from build123d import *

# Parameters (mm, degrees)
CYLINDER001_R          = 0.75
CYLINDER001_DEPTH      = 10
CYLINDER001_ROLL_ANGLE = 90
CYLINDER002_R          = 0.75
CYLINDER002_DEPTH      = 10
CYLINDER002_ROLL_ANGLE = 90
CYLINDER_R             = 15
CYLINDER_DEPTH         = 20
CYLINDER_ROLL_ANGLE    = 90
BOX001_W               = 8
BOX001_H               = 9
BOX001_DEPTH           = 40
BOX002_W               = 8
BOX002_H               = 9
BOX002_DEPTH           = 40
BOX_W                  = 120
BOX_H                  = 20
BOX_DEPTH              = 40


with BuildPart() as zylinder001:
    # Cylinder001 → Cylinder001 (new body)
    with BuildSketch(Plane.XY):
        Circle(CYLINDER001_R)
    extrude(amount=CYLINDER001_DEPTH)


with BuildPart() as zylinder001_1:
    # Cylinder001 roll: moved
    add(zylinder001.part.rotate(Axis((0, 0, 0), (1, 0, 0)), CYLINDER001_ROLL_ANGLE))


with BuildPart() as zylinder001_2:
    # Cylinder001 placement: moved
    add(zylinder001_1.part.moved(Location((0, 10, 20))))


with BuildPart() as zylinder002:
    # Cylinder002 → Cylinder002 (new body)
    with BuildSketch(Plane.XY):
        Circle(CYLINDER002_R)
    extrude(amount=CYLINDER002_DEPTH)


with BuildPart() as zylinder002_1:
    # Cylinder002 roll: moved
    add(zylinder002.part.rotate(Axis((0, 0, 0), (1, 0, 0)), CYLINDER002_ROLL_ANGLE))


with BuildPart() as zylinder002_2:
    # Cylinder002 placement: moved
    add(zylinder002_1.part.moved(Location((50, 10, 20))))


with BuildPart() as zylinder:
    # Cylinder → Cylinder (new body)
    with BuildSketch(Plane.XY):
        Circle(CYLINDER_R)
    extrude(amount=CYLINDER_DEPTH)


with BuildPart() as zylinder_1:
    # Cylinder roll: moved
    add(zylinder.part.rotate(Axis((0, 0, 0), (1, 0, 0)), CYLINDER_ROLL_ANGLE))


with BuildPart() as zylinder_2:
    # Cylinder placement: moved
    add(zylinder_1.part.moved(Location((25, 20, 20))))


with BuildPart() as fusion001:
    # Fusion001 base: copy of Zylinder
    add(zylinder_2.part)

    # Fusion001: union Zylinder001, Zylinder002
    add(zylinder001_2.part)
    add(zylinder002_2.part)


with BuildPart() as cube001:
    # Box001 → Box001 (new body)
    with BuildSketch(Plane(origin=(-1, 8, 0), x_dir=(1, 0, 0), z_dir=(0, 0, 1))):
        with Locations((4, 4.5)):
            Rectangle(BOX001_W, BOX001_H)
    extrude(amount=BOX001_DEPTH)


with BuildPart() as cube002:
    # Box002 → Box002 (new body)
    with BuildSketch(Plane(origin=(103, 8, 0), x_dir=(1, 0, 0), z_dir=(0, 0, 1))):
        with Locations((4, 4.5)):
            Rectangle(BOX002_W, BOX002_H)
    extrude(amount=BOX002_DEPTH)


with BuildPart() as fusion002:
    # Fusion base: copy of Zylinder
    add(zylinder_2.part)

    # Fusion: union Zylinder001, Zylinder002
    add(zylinder001_2.part)
    add(zylinder002_2.part)


with BuildPart() as fusion002_1:
    # Fusion placement: moved
    add(fusion002.part.moved(Location((60, 0, 0))))

    # Fusion002: union Fusion001, Cube001, Cube002
    add(fusion001.part)
    add(cube001.part)
    add(cube002.part)


with BuildPart() as motorhalterung:
    # Box → Box (new body)
    with BuildSketch(Plane(origin=(-5, 0, 0), x_dir=(1, 0, 0), z_dir=(0, 0, 1))):
        with Locations((60, 10)):
            Rectangle(BOX_W, BOX_H)
    extrude(amount=BOX_DEPTH)

    # Cut: cut Fusion002
    add(fusion002_1.part, mode=Mode.SUBTRACT)


solid = motorhalterung.part
Verification items for the finished model (mm, model axes). A direction names the side the tool comes from. Coordinates: 2 decimals unless noted, no trailing zeros. Loops run counter-clockwise (first coordinate to the right, second up) from the corner with the lowest first, then second, coordinate; pieces in that order, holes last. Notation, with made-up numbers: (-31.75, -30) -> (25.25, -30) arc R28 cw to (25.25, 7) -> close; hole circle Ø9 at (58, 81). An arc over 180 degrees is marked (long way). Answer as CSV lines item,"result".
1) Cross-section at B-B, the plane z = 25.5. Record the cut outline in (x, y), then the cut area to 3 significant figures.
Found:
outline,"(-5, 0) -> (11.04, 0) -> (11.04, 20) -> (-5, 20) -> close; (38.96, 0) -> (71.04, 0) -> (71.04, 20) -> (38.96, 20) -> close; (98.96, 0) -> (115, 0) -> (115, 20) -> (98.96, 20) -> close; hole (-1, 8) -> (7, 8) -> (7, 17) -> (-1, 17) -> close; hole (103, 8) -> (111, 8) -> (111, 17) -> (103, 17) -> close"
area,"1,140 mm2"
2) Thickness scan on L1, parallel to Z at x = 25, y = 9.75; L2, parallel to X at y = 4, z = 17; L3, parallel to X at y = 3, z = 16. Record the ranges inside material, lowest first. Write a range as from..to.
Found:
L1,"z = 0..5, 35..40"
L2,"x = -5..10.3, 39.7..70.3, 99.7..115"
L3,"x = -5..10.54, 39.46..70.54, 99.46..115"
3) Cross-section at A-A, the plane y = 12.75. Record the cut outline in (x, z), then the cut area to 3 significant figures.
Found:
outline,"(-5, 0) -> (-1, 0) -> (-1, 40) -> (-5, 40) -> close; (7, 0) -> (103, 0) -> (103, 40) -> (7, 40) -> close; (111, 0) -> (115, 0) -> (115, 40) -> (111, 40) -> close; hole circle Ø30 at (25, 20); hole circle Ø30 at (85, 20)"
area,"2,750 mm2"
4) Tool access check on faces 5 (the flat face through (3, 8, 20)), 6 (the flat face through (115, 10, 20)). Record the directions out of +Z, -Z, +X, -X, +Y, -Y that give a thin tool (end or side, any length) a straight path to the whole face; none if there is none.
Found:
face 5,"+Z, -Z"
face 6,"+Z, -Z, +X, +Y, -Y"
5) Cross-section at C-C, the plane x = 85. Record the cut outline in (y, z), then the cut area to 3 significant figures.
Found:
outline,"(0, 0) -> (20, 0) -> (20, 5) -> (0, 5) -> close; (0, 35) -> (20, 35) -> (20, 40) -> (0, 40) -> close"
area,"200 mm2"
6) Depth check by flat-ended pin: pin 1 (12 mm diameter, centred on x = 91.5, z = 16.5, fed in from +Y); pin 2 (0.9 mm diameter, centred on x = 60, z = 20, fed in from -Y). Enter the tip coordinate at first touch or a pass-through.
Found:
pin 1,"passes through"
pin 2,"stops at y = 10"
7) Cross-section at D-D, the plane y = 4.5. Record the cut outline in (x, z).
Found:
outline,"(-5, 0) -> (115, 0) -> (115, 40) -> (-5, 40) -> close; hole circle Ø1.5 at (0, 20); hole circle Ø30 at (25, 20); hole circle Ø1.5 at (50, 20); hole circle Ø1.5 at (60, 20); hole circle Ø30 at (85, 20); hole circle Ø1.5 at (110, 20)"
8) Release check for a two-part mould opening along Z. For faces 1 (the flat face through (54, 10, 40)), 2 (the cylindrical face through (21.748, 10.14, 5.357)), 3 (the flat face through (7, 12, 20)), 4 (the flat face through (54, 10, 0)) record: +Z half, -Z half, draft (parallel to the pull), parting line (faces both ways), or undercut.
Found:
face 1,"+Z half"
face 2,"undercut"
face 3,"draft"
face 4,"-Z half"
